from build123d import *

# Parameters (mm, degrees)
EXTRUDE1_DEPTH = 14
SKETCH2_W      = 7.8
SKETCH2_H      = 14
EXTRUDE2_DEPTH = 0.8
HOLEWZD1_D     = 4.917
HOLEWZD1_DEPTH = 6.3
CHAMFER1_SIZE  = 0.5415


with BuildPart() as part:
    # Sketch1 → Extrude1 (new body)
    with BuildSketch(Plane(origin=(0, 28.5, 0), x_dir=(1, 0, 0), z_dir=(0, 1, 0))):
        Polygon((11.6, 15.6), (8, 10.1), (23, 10.1), (19.4, 15.6), align=None)
    extrude(amount=-EXTRUDE1_DEPTH)

    # Sketch2 → Extrude2 (add)
    with BuildSketch(Plane.XY.offset(-10.1)):
        with Locations((15.5, 21.5)):
            Rectangle(SKETCH2_W, SKETCH2_H)
    extrude(amount=EXTRUDE2_DEPTH)

    # HoleWzd1
    with Locations(Plane.XY.offset(-9.3)):
        with Locations((15.5, 21.5)):
            Hole(HOLEWZD1_D / 2, depth=HOLEWZD1_DEPTH)

    # Chamfer1
    chamfer1_edges = [part.edges().sort_by_distance(p)[0] for p in [
        (17.9585, 21.5, -9.3),
        (17.9585, 21.5, -15.6),
    ]]
    chamfer(chamfer1_edges, length=CHAMFER1_SIZE)


solid = part.part
Build history of the part. All positions in model axes, mm. A direction names the side the tool comes from. Coordinates: 2 decimals unless noted, no trailing zeros. Order: outer loops, then holes, each group sorted by start corner. A loop starts at its lowest first (then second) coordinate and runs counter-clockwise, first axis right, second up. Notation, with made-up numbers: (24, 29.25) - (43, 29.25) arc R20 cw to (43, 63.25) - close; hole circle Ø1 at (53.25, -7.5). An arc over 180 degrees is marked (long way). Write each question's results on one line, items separated by ' | '. Start each with the question number.
Item 1: Band-saw the part on C-C on y = 24.75. Write the cut outline in (x, z).
Item 2: Band-saw the part on A-A on y = 21.5. Write the cut outline in (x, z), and give its area (3 significant figures).
Item 3: Band-saw the part on B-B on x = 15.5. Write the cut outline in (y, z).
Item 4: Band-saw the part on D-D on z = -12.5. Write the cut outline in (x, y).
Item 5: Wall check: probe 1 along Y at (x, z) = (15.5, -12.8); probe 2 along X at (y, z) = (22.25, -13); probe 3 along X at (y, z) = (19.5, -11.25). Give the ranges that are in metal, low to high. Write a range as [from, to].
Item 6: Flat gauge pins, fed straight in: pin 1 (0.6 mm diameter, centred on y = 20, z = -9.5, fed in from -X); pin 2 (1 mm diameter, centred on x = 20, y = 20.5, fed in from +Z); pin 3 (3 mm diameter, centred on y = 24.5, z = -14.5, fed in from +X); pin 4 (4 mm diameter, centred on x = 15.5, y = 21.5, fed in from -Z). Where does each tip first touch, or does it go through?
Item 7: Tool access for faces 1 (the face through (19.4, 21.4, -9.7)), 2 (the face through (18.2, 23.2, -15.6)), 3 (the face through (10, 22, -10.1)): list every direction of +Z, -Z, +X, -X, +Y, -Y with a clear straight run to the whole face (end or side of a thin tool).
Item 8: Mould opens along Y. For faces 4 (the face through (15, 28.5, -12)), 5 (the face through (9.825, 21.598, -12.888)), 6 (the face through (17.956, 21.608, -12.487)) say: released by +Y, released by -Y, zero draft, split by the parting line, or undercut.
Numbers:
1) outline: (8, -10.1) - (11.6, -15.6) - (19.4, -15.6) - (23, -10.1) - (19.4, -10.1) - (19.4, -9.3) - (11.6, -9.3) - (11.6, -10.1) - close
2) outline: (8, -10.1) - (11.6, -15.6) - (12.5, -15.6) - (13.04, -15.06) - (13.04, -9.84) - (12.5, -9.3) - (11.6, -9.3) - (11.6, -10.1) - close; (17.96, -15.06) - (18.5, -15.6) - (19.4, -15.6) - (23, -10.1) - (19.4, -10.1) - (19.4, -9.3) - (18.5, -9.3) - (17.96, -9.84) - close | area: 37.4 mm^2
3) outline: (14.5, -15.6) - (18.5, -15.6) - (19.04, -15.06) - (19.04, -9.84) - (18.5, -9.3) - (14.5, -9.3) - close; (23.96, -15.06) - (24.5, -15.6) - (28.5, -15.6) - (28.5, -9.3) - (24.5, -9.3) - (23.96, -9.84) - close
4) outline: (9.57, 14.5) - (21.43, 14.5) - (21.43, 28.5) - (9.57, 28.5) - close; hole circle Ø4.92 at (15.5, 21.5)
5) probe 1: [14.5, 19.04], [23.96, 28.5] | probe 2: [9.9, 13.16], [17.84, 21.1] | probe 3: [8.75, 14.07], [16.93, 22.25]
6) pin 1: x = 11.6 | pin 2: z = -10.1 | pin 3: x = 21.1 | pin 4: through
7) face 1: +Z, +X, +Y, -Y | face 2: -Z, +X, -X, +Y, -Y | face 3: +Z, -X, +Y, -Y
8) face 4: released by +Y | face 5: zero draft | face 6: undercut
